```python
from build123d import *

# Parameters (mm, degrees)
F3_ANGLE = 90
F5_ANGLE = 90


with BuildPart() as f1:
    # F0 (on Front) → F1 (revolve)
    with BuildSketch(Plane.XZ):
        with BuildLine():
            Line((-21, 16.5), (-26, 16.5))
            ThreePointArc((-26, 16.5), (-27.5, 15), (-26, 13.5))
            Line((-26, 13.5), (-21, 13.5))
            Line((-21, 13.5), (-21, 16.5))
        make_face()
    revolve(axis=Axis((0, 0, 12.5856157392), (0, 0, -1)))

    # F2 (on Front) → F3 (revolve)
    with BuildSketch(Plane.XZ):
        with BuildLine():
            Line((-22.8234108924, 15.5310801728), (-20.9705103189, 13.5594885796))
            Line((-20.9705103189, 13.5594885796), (-18.0268532264, 16.3259357148))
            add(Edge.make_bspline(
                [(-18.0268532264, 16.3259357148), (2.5248612882, 21.0512280006), (-3.0509901699, 30.4002426565)],
                knots=[4.0760424662, 4.0760424662, 4.0760424662, 6.2831853072, 6.2831853072, 6.2831853072], degree=2, weights=[1, 0.4504103592, 1]))
            Line((-3.0509901699, 30.4002426565), (-3.7834591359, 31.1796312952))
            Line((-3.7834591359, 31.1796312952), (-4.9038907434, 32.3718342497))
            Line((-4.9038907434, 32.3718342497), (-22.8234108924, 15.5310801728))
        make_face()
        with BuildLine():
            Line((-3.7834591359, 31.1796312952), (-3.0509901699, 30.4002426565))
            add(Edge.make_bspline(
                [(-3.0509901699, 30.4002426565), (-3.3209830741, 30.8529390092), (-3.7834591359, 31.1796312952)],
                knots=[0, 0, 0, 0.1913811194, 0.1913811194, 0.1913811194], degree=2, weights=[1, 0.9954251509, 1]))
        make_face()
    revolve(axis=Axis((0, 0, 24.1673644632), (0, 0, -1)), revolution_arc=F3_ANGLE)

    # F4 (on Front) → F5 (revolve)
    with BuildSketch(Plane.XZ):
        with BuildLine():
            Line((-4.9122721049, 32.3865450188), (-6.1626020759, 31.2069066763))
            Line((-6.1626020759, 31.2069066763), (-6.1446281649, 31.1877814126))
            add(Edge.make_bspline(
                [(-18.9718568385, 17.0376612359), (-14.9669974913, 17.146964893), (-9.6910325347, 22.9670480991), (-4.4150675782, 28.7871313051), (-6.1446281649, 31.1877814126)],
                knots=[3.5205813128, 3.5205813128, 3.5205813128, 4.8740420257, 4.8740420257, 6.2275027386, 6.2275027386, 6.2275027386], degree=2, weights=[1, 0.7796244878, 1, 0.7796244878, 1]))
            Line((-18.9718568385, 17.0376612359), (-21.7830147594, 16.4930532639))
            Line((-21.7830147594, 16.4930532639), (-21.7830147594, 16.4715316409))
            add(Edge.make_bspline(
                [(-21.7830147594, 16.4715316409), (-17.9606831235, 12.4873048362), (-9.5363391364, 20.4118410334), (-1.1119951493, 28.3363772305), (-4.8897280053, 32.3625568147)],
                knots=[0.0052940421, 0.0052940421, 0.0052940421, 1.5734433479, 1.5734433479, 3.1415926536, 3.1415926536, 3.1415926536], degree=2, weights=[1, 0.7080420249, 1, 0.7080420249, 1]))
            Line((-4.8897280053, 32.3625568147), (-4.9122721049, 32.3865450188))
        make_face()
    revolve(axis=Axis((0, 0, 25.1945196651), (0, 0, 1)), revolution_arc=F5_ANGLE)


solid = f1.part
```
Work out the finished part from the listing and answer in its coordinate system (mm). A direction names the side the tool comes from. Give positions to 0.01 mm unless a question says otherwise; leave off trailing zeros.
1. The mould has two halves that part along X. Classify faces 1 (the flat face through (21, -4, 16.5)), 2 (the cylindrical face through (16.665, -12.778, 15.021)), 3 (the conical face through (-13.7, -13.4, 17)): released by +X, released by -X, zero draft, split by the parting line, or undercut.
Result sheet:
face 1: zero draft
face 2: undercut
face 3: released by -X
2. Straight lines are drawn through the part: L1, parallel to X at y = -15, z = 15; L2, parallel to Y at x = -1, z = 25; L3, parallel to Z at x = -19.5, y = -11.5. For each, find the intervals that lie inside material, in ascending order.
Result sheet:
L1: x = -23.05 to -14.7, 14.7 to 23.05
L2: y = -7.97 to -5.69, 4.24 to 12.71
L3: z = 13.5 to 16.5
3. Each of these flat-tipped pins is pushed along its axis until it touches: P1, Ø8.5, axis at x = -8, z = 27.5, coming from the -Y side; P2, Ø1.2, axis at x = -16.5, z = 18, coming from the +Y side; P3, Ø12, axis at x = -17.5, y = -19.5, coming from the +Z side. Where does it stop, or does it pass through?
Result sheet:
P1: stops at y = -6.81
P2: stops at y = 12.97
P3: stops at z = 16.8
4. For faces 4 (the conical face through (-3.77, -3.68, 32.05)), 5 (the flat face through (-20, 0, 15)), 6 (the conical face through (-2.93, 2.87, 31.52)), determine the directions among +Z, -Z, +X, -X, +Y, -Y from which every point of the face is accessible in a straight line to the end or side of a thin tool.
Result sheet:
face 4: +Z, -X, -Y
face 5: -Z
face 6: +Z, +X
